```python
from build123d import *

# Parameters (mm, degrees)
BOSS_EXTRU_2_DEPTH      = 120
ESQUISSE2_R             = 2.25
ENL_V_MAT_EXTRU_1_DEPTH = 5
ESQUISSE4_W             = 78
ESQUISSE4_H             = 52
BOSS_EXTRU_3_DEPTH      = 4
ESQUISSE6_R             = 5
ENL_V_MAT_EXTRU_3_DEPTH = 10


with BuildPart() as part:
    # Esquisse1 → Boss.-Extru.2 (new body)
    with BuildSketch(Plane(origin=(0, 0, 0), x_dir=(1, 0, 0), z_dir=(0, 1, 0))):
        Polygon((71, -60), (78, -60), (78, 0), (0, 0), (0, -60), (7, -60), (7, -57), (4, -57), (4, -10), (14, -10), (14, -4), (64, -4), (64, -10), (74, -10), (74, -57), (71, -57), align=None)
    extrude(amount=BOSS_EXTRU_2_DEPTH)

    # Esquisse2 → Enlèv. mat.-Extru.1 (cut)
    with BuildSketch(Plane.XZ):
        with Locations((69, 5)):
            Circle(ESQUISSE2_R)
        with Locations((9, 5)):
            Circle(ESQUISSE2_R)
    extrude(amount=-ENL_V_MAT_EXTRU_1_DEPTH, mode=Mode.SUBTRACT)

    # Esquisse4 → Boss.-Extru.3 (add)
    with BuildSketch(Plane(origin=(0, 120, 0), x_dir=(1, 0, 0), z_dir=(0, 1, 0))):
        with Locations((39, -26)):
            Rectangle(ESQUISSE4_W, ESQUISSE4_H)
    extrude(amount=BOSS_EXTRU_3_DEPTH)

    # Esquisse6 → Enlèv. mat.-Extru.3 (cut)
    with BuildSketch(Plane(origin=(0, 124, 0), x_dir=(1, 0, 0), z_dir=(0, 1, 0))):
        with Locations((15, -30)):
            Circle(ESQUISSE6_R)
        with Locations((63, -30)):
            Circle(ESQUISSE6_R)
    extrude(amount=-ENL_V_MAT_EXTRU_3_DEPTH, mode=Mode.SUBTRACT)


solid = part.part
```
CAD build for the part. Positions are in the model's coordinates, mm. A direction names the side the tool comes from. Round coordinates to 2 decimals unless told otherwise and drop trailing zeros. Write each loop counter-clockwise with the first axis right and the second up, starting at its lowest first coordinate (ties: lowest second). Pieces come first, ordered by that corner, then holes. Notation, with made-up numbers: M 16.5,54.25 L 45.5,54.25 A19 ccw 45.5,59.25 Z; hole C -21,78.5 d2. An arc over 180 degrees is marked long. One line per question, with ' | ' between items.
1. Cut at B-B on y = 37.5. Write the cut outline in (x, z).
Working result:
outline: M 0,0 L 78,0 L 78,60 L 71,60 L 71,57 L 74,57 L 74,10 L 64,10 L 64,4 L 14,4 L 14,10 L 4,10 L 4,57 L 7,57 L 7,60 L 0,60 Z
2. Which spindle directions (+Z, -Z, +X, -X, +Y, -Y) get a long thin tool onto all of the face, cutting with end or side? Do faces 1 (the flat face through (9, 5, 5)), 2 (the flat face through (73, 59, 57)), 3 (the flat face through (38, 61, 0)), 4 (the flat face through (39, 59, 4)), 5 (the flat face through (71, 59, 58)). Say none if no direction does.
Working result:
face 1: -Y | face 2: +Y, -Y | face 3: -Z, +X, -X, +Y, -Y | face 4: +Z, -Y | face 5: +Z, +Y, -Y
3. Pin check, flat tips, straight feed: pin 1 Ø3.5 at (x, z) = (3.5, 56.5) entering from +Y; pin 2 Ø6 at (x, y) = (63, 73) entering from +Z; pin 3 Ø2.5 at (x, z) = (69, 5) entering from -Y. Stop position of each tip, or through.
Working result:
pin 1: y = 120 | pin 2: z = 10 | pin 3: y = 5
4. Mould opens along X. For faces 6 (the flat face through (78, 61, 30)), 7 (the flat face through (74, 59, 60)), 8 (the flat face through (69, 59, 10)), 9 (the flat face through (0, 61, 30)) say: pulls with the +X half, pulls with the -X half, needs draft (parallel to the pull), parting line crosses it, or undercut.
Working result:
face 6: pulls with the +X half | face 7: needs draft | face 8: undercut | face 9: pulls with the -X half
5. Cut at C-C on z = 20. Write the cut outline in (x, y).
Working result:
outline: M 0,0 L 4,0 L 4,120 L 74,120 L 74,0 L 78,0 L 78,124 L 0,124 Z
6. Probe L1, parallel to X at y = 122, z = 30; L2, parallel to X at y = 44, z = 47; L3, parallel to Z at x = 73, y = 114.5. List the from-to ranges inside material, lowest first. Write a range as from..to.
Working result:
L1: 0..10, 20..58, 68..78 | L2: 0..4, 74..78 | L3: 0..10, 57..60
7. Cut at A-A on z = 30. Write the cut outline in (x, y).
Working result:
outline: M 0,0 L 4,0 L 4,120 L 10,120 L 10,124 L 0,124 Z; M 20,120 L 58,120 L 58,124 L 20,124 Z; M 68,120 L 74,120 L 74,0 L 78,0 L 78,124 L 68,124 Z
